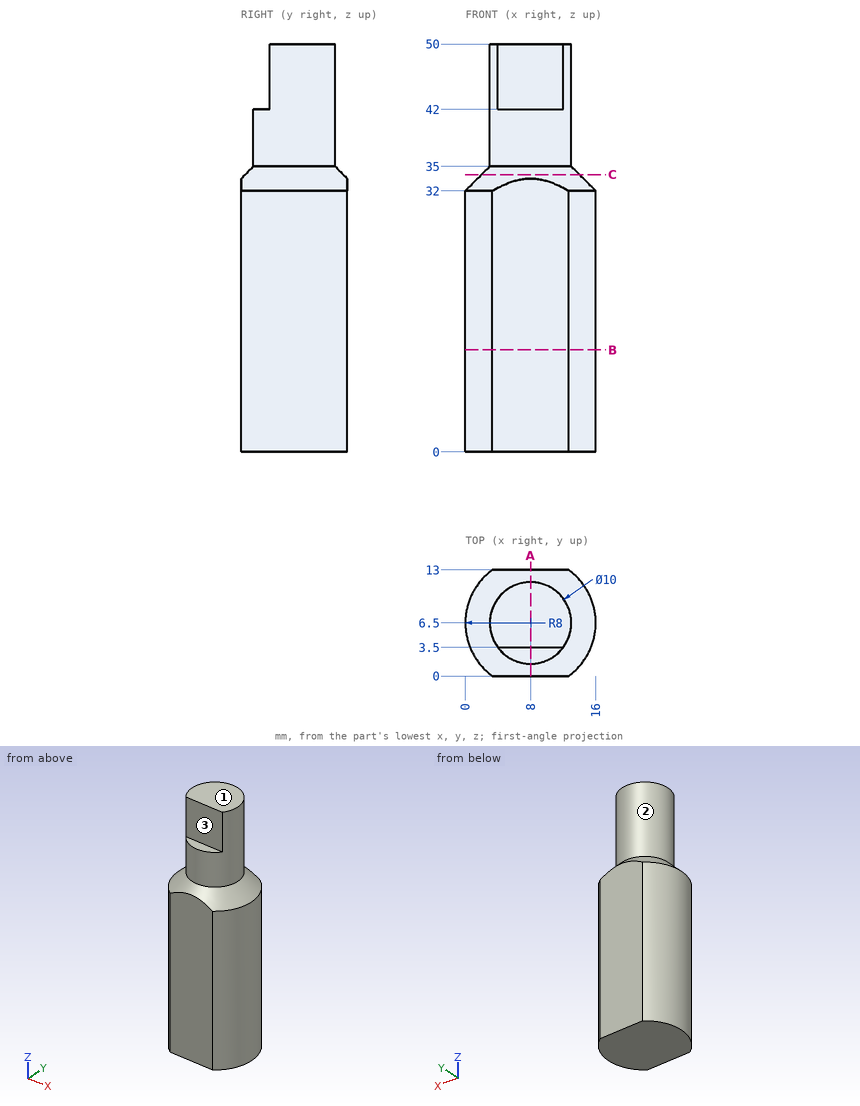
Geometry: see drawing. Coordinates: mm, zero at the bounding-box minimum. A direction names the side the tool comes from. Coordinates: 2 decimals unless noted, no trailing zeros. Loops run counter-clockwise (first coordinate to the right, second up) from the corner with the lowest first, then second, coordinate; pieces in that order, holes last.
Q1. Material intervals for line 1 (X direction, y = 6.75, z = 32.5); line 2 (Z direction, x = 4, y = 1); line 3 (Y direction, x = 10.5, z = 34.5), sorted ascending.
Q2. Cut plane B-B (z = 12.5). Output: boundary loops of the cut face in (x, y), then the cut area to 3 significant figures.
Q3. Contact query for flat-ended pins moving along their axis: pin 1 (2 mm diameter, centred on y = 4.5, z = 27.5, fed in from +X); pin 2 (2.5 mm diameter, centred on x = 6, z = 45, fed in from -Y); pin 3 (4 mm diameter, centred on x = 3, y = 1.5, fed in from +Z); pin 4 (3 mm diameter, centred on x = 7.5, y = 1.5, fed in from -Z). Output: stop coordinate, or through.
Q4. Cut plane C-C (z = 34). Output: boundary loops of the cut face in (x, y), then the cut area to 3 significant figures.
Q5. Set-up query: the marked faces 1, 2 and 3. Return all of +Z, -Z, +X, -X, +Y, -Y with unobstructed straight access to the full face (end or side cutting, diameter ignored); none if empty.
Q6. Cut plane A-A (x = 8). Output: boundary loops of the cut face in (y, z), then the cut area to 3 significant figures.
Working result:
1. line 1: x = 0.5 to 15.5
1. line 2: z = 0 to 33.2
1. line 3: y = 1.6 to 11.4
2. outline: (3.34, 0) - (12.66, 0) arc R8 ccw to (12.66, 13) - (3.34, 13) arc R8 ccw to start
2. area: 182 mm2
3. pin 1: stops at x = 15.94
3. pin 2: stops at y = 3.5
3. pin 3: stops at z = 34.93
3. pin 4: stops at z = 0
4. outline: circle Ø12 at (8, 6.5)
4. area: 113 mm2
5. face 1: +Z, +X, -X, +Y, -Y
5. face 2: +Z
5. face 3: +Z, +X, -X, -Y
6. outline: (0, 0) - (13, 0) - (13, 33.5) - (11.5, 35) - (11.5, 50) - (3.5, 50) - (3.5, 42) - (1.5, 42) - (1.5, 35) - (0, 33.5) - close
6. area: 587 mm2
